```python
from build123d import *

# Parameters (mm, degrees)
EXTRUDE_1_DEPTH      = 25
CUT_EXTRUDE_4_DEPTH  = 80.457942189
SKETCH_7_W           = 16.60831278
SKETCH_7_H           = 38.473598513
CUT_EXTRUDE_14_DEPTH = 80.457942189
SKETCH_8_W           = 5
SKETCH_8_H           = 30.968526609
EXTRUDE_2_DEPTH      = 25
SKETCH_9_W           = 2.765387297
SKETCH_9_H           = 65
EXTRUDE_3_DEPTH      = 100
SKETCH_10_W          = 5.026813651
SKETCH_10_H          = 30.968526609
EXTRUDE_4_DEPTH      = 40
CUT_EXTRUDE_15_DEPTH = 100
SKETCH_12_R          = 28.5
CUT_EXTRUDE_16_DEPTH = 100
SKETCH_13_R          = 1.25
CUT_EXTRUDE_17_DEPTH = 100
CHAMFER_1_SIZE       = 10


with BuildPart() as part:
    # Эскиз1 → Бобышка-Вытянуть1 (new body)
    with BuildSketch(Plane(origin=(0, 0, 0), x_dir=(1, 0, 0), z_dir=(0, 1, 0))):
        Polygon((-66.825757576, 34.969739794), (-66.825757576, 29.969739794), (-63.825757576, 29.969739794), (-63.825757576, 31.969739794), (-38.825757576, 31.969739794), (-38.825757576, 6.969739794), (-63.825757576, 6.969739794), (-63.825757576, 8.969739794), (-66.825757576, 8.969739794), (-66.825757576, 3.969739794), (-22.123470102, 3.969739794), (-36.579007505, 34.969739794), align=None)
    extrude(amount=EXTRUDE_1_DEPTH)

    # Эскиз3 → Вырез-Вытянуть4 (cut, through all)
    with BuildSketch(Plane.XZ):
        Polygon((-66.825757576, -3.969739794), (-65.325757576, -8.969739794), (-66.825757576, -8.969739794), align=None)
        Polygon((-66.825757576, -29.969739794), (-66.825757576, -34.969739794), (-65.325757576, -29.969739794), align=None)
    extrude(amount=-CUT_EXTRUDE_4_DEPTH, mode=Mode.SUBTRACT)

    # Эскиз7 → Вырез-Вытянуть14 (cut, through all)
    with BuildSketch(Plane(origin=(0, 0, 0), x_dir=(-1, 0, 0), z_dir=(0, -1, 0))):
        with Locations((27.703474463, 20.539743139)):
            Rectangle(SKETCH_7_W, SKETCH_7_H)
    extrude(amount=-CUT_EXTRUDE_14_DEPTH, mode=Mode.SUBTRACT)

    # Эскиз8 → Бобышка-Вытянуть2 (add)
    with BuildSketch(Plane(origin=(0, 0, 0), x_dir=(-1, 0, 0), z_dir=(0, -1, 0))):
        with Locations((36.298943925, 19.454003098)):
            Rectangle(SKETCH_8_W, SKETCH_8_H)
    extrude(amount=-EXTRUDE_2_DEPTH)

    # Эскиз9 → Бобышка-Вытянуть3 (add)
    with BuildSketch(Plane(origin=(0, 0, -34.938266403), x_dir=(-1, 0, 0), z_dir=(0, 0, -1))):
        with Locations((38.181637573, 32.5)):
            Rectangle(SKETCH_9_W, SKETCH_9_H)
    extrude(amount=EXTRUDE_3_DEPTH)

    # Эскиз10 → Бобышка-Вытянуть4 (add)
    with BuildSketch(Plane(origin=(0, 25, 0), x_dir=(1, 0, 0), z_dir=(0, 1, 0))):
        with Locations((-36.312350751, 19.454003098)):
            Rectangle(SKETCH_10_W, SKETCH_10_H)
    extrude(amount=EXTRUDE_4_DEPTH)

    # Эскиз11 → Вырез-Вытянуть15 (cut)
    with BuildSketch(Plane(origin=(-33.798943925, 0, 0), x_dir=(0, 0, -1), z_dir=(1, 0, 0))):
        Polygon((34.938266403, 65), (3.969739794, 32.5), (3.969739794, 65), align=None)
    extrude(amount=-CUT_EXTRUDE_15_DEPTH, mode=Mode.SUBTRACT)

    # Эскиз12 → Вырез-Вытянуть16 (cut)
    with BuildSketch(Plane(origin=(-36.798943925, 0, 0), x_dir=(0, 0, -1), z_dir=(1, 0, 0))):
        with Locations((102.438266403, 32.5)):
            Circle(SKETCH_12_R)
    extrude(amount=-CUT_EXTRUDE_16_DEPTH, mode=Mode.SUBTRACT)

    # Эскиз13 → Вырез-Вытянуть17 (cut)
    with BuildSketch(Plane(origin=(-36.798943925, 0, 0), x_dir=(0, 0, -1), z_dir=(1, 0, 0))):
        with Locations((77.438266403, 57.5)):
            Circle(SKETCH_13_R)
        with Locations((127.438266403, 57.5)):
            Circle(SKETCH_13_R)
        with Locations((127.438266403, 7.5)):
            Circle(SKETCH_13_R)
        with Locations((77.438266403, 7.5)):
            Circle(SKETCH_13_R)
    extrude(amount=-CUT_EXTRUDE_17_DEPTH, mode=Mode.SUBTRACT)

    # Фаска1
    chamfer_1_edges = [part.edges().sort_by_distance(p)[0] for p in [
        (-39.564331222, 12.5, -34.969739794),
    ]]
    chamfer(chamfer_1_edges, length=CHAMFER_1_SIZE)


solid = part.part
```
Work out the finished part from the listing and answer in its coordinate system (mm). A direction names the side the tool comes from. Coordinates: 2 decimals unless noted, no trailing zeros. Loops run counter-clockwise (first coordinate to the right, second up) from the corner with the lowest first, then second, coordinate; pieces in that order, holes last.
1) Consider probe 1 along Z at (x, y) = (-38, 32); probe 2 along Z at (x, y) = (-38, 7); probe 3 along X at (y, z) = (35.5, -12). Determine where each line is inside the solid, lowest interval first.
Results:
probe 1: z = -134.94 to -130.93, -73.94 to -3.97
probe 2: z = -134.94 to -128.58, -126.29 to -115.17, -89.71 to -78.58, -76.29 to -3.97
probe 3: x = -38.83 to -33.8
2) Section C-C (x = -42) is taken. Give the vertices of the cut face in (y, z).
Results:
outline: (0, -42.53) - (25, -42.53) - (25, -31.97) - (0, -31.97) - close; (0, -6.97) - (25, -6.97) - (25, -3.97) - (0, -3.97) - close
3) Section B-B (y = 7.5) is taken. Give the number of separate pieces and of enclosed holes in the cut face, plus the area to 3 significant figures.
Results:
separate pieces: 4
enclosed holes: 0
area: 565 mm2
4) Section D-D (z = -114) is taken. Give the vertices of the cut face in (x, y), plus the area to 3 significant figures.
Results:
outline: (-39.56, 0) - (-36.8, 0) - (-36.8, 6.45) - (-39.56, 6.45) - close; (-39.56, 58.55) - (-36.8, 58.55) - (-36.8, 65) - (-39.56, 65) - close
area: 35.7 mm2
5) Flat-ended cylindrical pins translate along their axes: pin 1 (1.5 mm diameter, centred on x = -53, z = -7, fed in from +Y); pin 2 (6 mm diameter, centred on y = 53.5, z = -81, fed in from +X); pin 3 (12 mm diameter, centred on x = -51.5, z = -76.5, fed in from +Y); pin 4 (6 mm diameter, centred on y = 23, z = -68, fed in from -X). Find the tip coordinate at first contact, or state that the pin passes through.
Results:
pin 1: stops at y = 25
pin 2: stops at x = -36.8
pin 3: passes through
pin 4: stops at x = -39.56
6) For faces 4 (the cylindrical face through (-38.16, 51.76, -81.43)), 5 (the flat face through (-52, 12, -31.97)), 6 (the flat face through (-51, 12, -3.97)), 7 (the flat face through (-66.086, 12.325, -32.505)), 8 (the flat face through (-58, 12, -34.97)), determine the directions among +Z, -Z, +X, -X, +Y, -Y from which every point of the face is accessible in a straight line to the end or side of a thin tool.
Results:
face 4: +X, -X
face 5: +Y, -Y
face 6: +Z, +X, -X, +Y, -Y
face 7: -X, +Y, -Y
face 8: -Z, -X, +Y, -Y
7) Section A-A (y = 36) is taken. Give the vertices of the cut face in (x, z).
Results:
outline: (-39.56, -134.94) - (-36.8, -134.94) - (-36.8, -130.72) - (-39.56, -130.72) - close; (-39.56, -74.15) - (-36.8, -74.15) - (-36.8, -34.94) - (-33.8, -34.94) - (-33.8, -7.3) - (-38.83, -7.3) - (-38.83, -34.94) - (-39.56, -34.94) - close
8) For a pull along X with two mould halves and no side action, classify faces 1 (the flat face through (-66.086, 12.325, -6.435)), 2 (the flat face through (-51, 12, -6.97)), 3 (the flat face through (-36.799, 32, -73)) as +X half, -X half, draft (parallel to the pull), parting line (faces both ways), or undercut.
Results:
face 1: -X half
face 2: undercut
face 3: +X half
